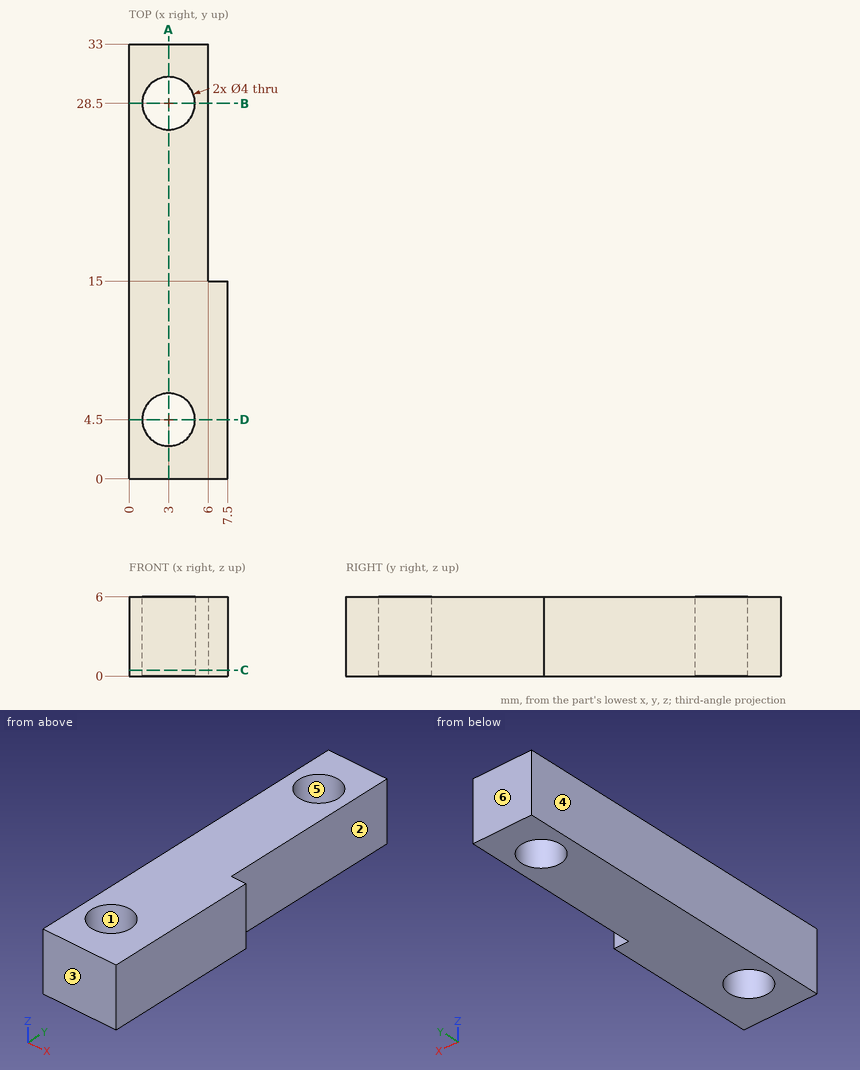
Answer from the drawing. Dimensions are ordinates in mm from the lowest x, y and z of the part. A direction names the side the tool comes from. Coordinates: 2 decimals unless noted, no trailing zeros. Order: outer loops, then holes, each group sorted by start corner. A loop starts at its lowest first (then second) coordinate and runs counter-clockwise, first axis right, second up. Notation, with made-up numbers: (36.5, 37) - (74.5, 37) arc R15 ccw to (74.5, 63) - close; hole circle Ø9 at (-9.5, 89.5). An arc over 180 degrees is marked (long way). Use one line per item in the form item = value.
(1) Given pin 1 Ø3.5 at (x, y) = (3, 28.5) entering from -Z, flat-ended and moving along its own axis, determine where the tip first touches the part or whether it passes through.
Computed values:
pin_1 = through
(2) Section A-A, the plane x = 3 is taken. Give the vertices of the cut face in (y, z), then the cut area to 3 significant figures.
Computed values:
outline = (0, 0) - (2.5, 0) - (2.5, 6) - (0, 6) - close; (6.5, 0) - (26.5, 0) - (26.5, 6) - (6.5, 6) - close; (30.5, 0) - (33, 0) - (33, 6) - (30.5, 6) - close
area = 150 mm²
(3) Section B-B, the plane y = 28.5 is taken. Give the vertices of the cut face in (x, z).
Computed values:
outline = (0, 0) - (1, 0) - (1, 6) - (0, 6) - close; (5, 0) - (6, 0) - (6, 6) - (5, 6) - close
(4) For a pull along Y with two mould halves and no side action, classify the marked faces 3, 4, 5 and 6 as pulls with the +Y half, pulls with the -Y half, needs draft (parallel to the pull), parting line crosses it, or undercut.
Computed values:
face_3 = pulls with the -Y half
face_4 = needs draft
face_5 = undercut
face_6 = pulls with the +Y half
(5) Section D-D, the plane y = 4.5 is taken. Give the vertices of the cut face in (x, z), then the cut area to 3 significant figures.
Computed values:
outline = (0, 0) - (1, 0) - (1, 6) - (0, 6) - close; (5, 0) - (7.5, 0) - (7.5, 6) - (5, 6) - close
area = 21.0 mm²
(6) Which of the six approach directions +Z, -Z, +X, -X, +Y, -Y give full straight-line access (tool end or side, diameter ignored) to the marked faces 1 and 2?
Computed values:
face_1 = +Z, -Z
face_2 = +Z, -Z, +X, +Y
(7) Section C-C, the plane z = 0.45 is taken. Give the vertices of the cut face in (x, y), then the cut area to 3 significant figures.
Computed values:
outline = (0, 0) - (7.5, 0) - (7.5, 15) - (6, 15) - (6, 33) - (0, 33) - close; hole circle Ø4 at (3, 4.5); hole circle Ø4 at (3, 28.5)
area = 195 mm²
(8) Straight lines are drawn through the part: L1, parallel to Y at x = 3, z = 2.75; L2, parallel to Y at x = 4.5, z = 2.55; L3, parallel to X at y = 16.5, z = 0.6. For each, find the intervals that lie inside material, in ascending order.
Computed values:
L1 = 0 to 2.5, 6.5 to 26.5, 30.5 to 33
L2 = 0 to 3.18, 5.82 to 27.18, 29.82 to 33
L3 = 0 to 6
